The model under review builds one solid part; all positions refer to its coordinate system, in mm. Round coordinates to 2 decimals unless told otherwise and drop trailing zeros. Order: outer loops, then holes, each group sorted by start corner. A loop starts at its lowest first (then second) coordinate and runs counter-clockwise, first axis right, second up. Notation, with made-up numbers: M 74,-39.75 L 92,-39.75 A15 ccw 92,-25.75 Z; hole C 39,-12.5 d8. An arc over 180 degrees is marked long. One line per item, written item: value. Start each with the question number.
from build123d import *
from build123d.topology import SkipClean

# Parameters (mm, degrees)
SKETCH1_R                     = 10.5
SKETCH1_W                     = 8
SKETCH1_H                     = 40
SKETCH1_R_2                   = 5
BOSS_EXTRUDE1_DEPTH           = 3
CUT_EXTRUDE1_REACH            = 140.687
SKETCH2_R                     = 2
BOSS_EXTRUDE2_DEPTH           = 3
SKETCH5_R                     = 2
CUT_EXTRUDE2_DEPTH            = 10
BOSS_EXTRUDE4_START           = -3
BOSS_EXTRUDE4_DEPTH           = 3
BOSS_EXTRUDE5_START           = -3
SKETCH8_R                     = 65
SKETCH8_R_2                   = 10.5
BOSS_EXTRUDE5_DEPTH           = 3
CUT_EXTRUDE4_START            = -10
CUT_EXTRUDE4_DEPTH            = 10
CUT_EXTRUDE6_REACH            = 237.869
SKETCH11_R                    = 2
CUT_EXTRUDE7_REACH            = 237.869
SKETCH12_R                    = 2
CSK_FOR_M3_SFHCS1_D           = 3.4
CSK_FOR_M3_SFHCS1_DEPTH       = 11.3
CSK_FOR_M3_SFHCS1_CSINK_D     = 6.72
CSK_FOR_M3_SFHCS1_CSINK_ANGLE = 90
CSK_FOR_M3_SFHCS1_TIP         = 1.021463052
CSK_FOR_M4_SFHCS1_D           = 4.5
CSK_FOR_M4_SFHCS1_DEPTH       = 11.3
CSK_FOR_M4_SFHCS1_CSINK_D     = 8.96
CSK_FOR_M4_SFHCS1_CSINK_ANGLE = 90
CSK_FOR_M4_SFHCS1_TIP         = 1.351936393
CSK_FOR_M3_SFHCS2_D           = 3.4
CSK_FOR_M3_SFHCS2_DEPTH       = 11.3
CSK_FOR_M3_SFHCS2_CSINK_D     = 6.72
CSK_FOR_M3_SFHCS2_CSINK_ANGLE = 90
CSK_FOR_M3_SFHCS2_TIP         = 1.021463052
CSK_FOR_M4_SFHCS2_D           = 4.5
CSK_FOR_M4_SFHCS2_DEPTH       = 11.3
CSK_FOR_M4_SFHCS2_CSINK_D     = 8.96
CSK_FOR_M4_SFHCS2_CSINK_ANGLE = 90
CSK_FOR_M4_SFHCS2_TIP         = 1.351936393
CUT_EXTRUDE8_REACH            = 237.869
SKETCH23_R                    = 1.5
CSK_FOR_M3_SFHCS3_D           = 3.4
CSK_FOR_M3_SFHCS3_DEPTH       = 11.3
CSK_FOR_M3_SFHCS3_CSINK_D     = 6.72
CSK_FOR_M3_SFHCS3_CSINK_ANGLE = 90
CSK_FOR_M3_SFHCS3_TIP         = 1.021463052


with BuildPart() as part:
    # Sketch1 → Boss-Extrude1 (new body)
    # profile 1 of 2: a face of its own
    with BuildSketch(Plane.XY):
        with BuildLine():
            ThreePointArc((-60, 0), (-52.867640737, 28.372743309), (-33.166247904, 50))
            Line((-33.166247904, 50), (-60, 50))
            Line((-60, 50), (-60, 0))
        make_face()
    # profile 2 of 2: a face of its own
    with BuildSketch(Plane.XY):
        with BuildLine():
            ThreePointArc((0, 60), (-17.320508076, 57.445626465), (-33.166247904, 50))
            ThreePointArc((-33.166247904, 50), (-52.867640737, 28.372743309), (-60, 0))
            ThreePointArc((-60, 0), (-15.529142706, -57.955549577), (51.961524227, -30))
            Line((51.961524227, -30), (56.882127578, -30))
            Line((56.882127578, -30), (90, -30))
            Line((90, -30), (90, -10.355339059))
            Line((90, -10.355339059), (117.67766953, 17.32233047))
            ThreePointArc((117.67766953, 17.32233047), (123.096988313, 44.567085809), (100, 60))
            Line((100, 60), (0, 60))
        make_face()
        Circle(SKETCH1_R, mode=Mode.SUBTRACT)
        with Locations((76, 0)):
            Rectangle(SKETCH1_W, SKETCH1_H, mode=Mode.SUBTRACT)
        with Locations((100, 35)):
            Circle(SKETCH1_R_2, mode=Mode.SUBTRACT)
    extrude(amount=BOSS_EXTRUDE1_DEPTH)

    # Sketch2 → Cut-Extrude1 (cut, up to next)
    with BuildSketch(Plane.XY.offset(3), mode=Mode.PRIVATE) as cut_extrude1_sk1:
        with Locations((60, 45)):
            Circle(SKETCH2_R)
    cut_extrude1_tool1 = extrude(cut_extrude1_sk1.sketch, amount=-CUT_EXTRUDE1_REACH, mode=Mode.PRIVATE) & part.part
    add(cut_extrude1_tool1.solids().sort_by_distance((60, 45, 3))[0], mode=Mode.SUBTRACT)

    # Sketch3 → Boss-Extrude2 (add)
    with BuildSketch(Plane(origin=(0, 0, 0), x_dir=(-1, 0, 0), z_dir=(0, 0, -1))):
        with BuildLine():
            Line((-30, 80), (-30, 60))
            Line((-30, 60), (0, 60))
            ThreePointArc((0, 60), (2.502176759, 59.947803225), (5, 59.791303716))
            Line((5, 59.791303716), (5, 80))
            Line((5, 80), (-30, 80))
        make_face()
    extrude(amount=-BOSS_EXTRUDE2_DEPTH)

    # Sketch5 → Cut-Extrude2 (cut)
    with BuildSketch(Plane.XY.offset(3)):
        with Locations((92, 43)):
            Circle(SKETCH5_R)
        with Locations((108, 43)):
            Circle(SKETCH5_R)
        with Locations((108, 27)):
            Circle(SKETCH5_R)
        with Locations((92, 27)):
            Circle(SKETCH5_R)
    extrude(amount=-CUT_EXTRUDE2_DEPTH, mode=Mode.SUBTRACT)

    # Sketch6 → Boss-Extrude4 (add)
    with BuildSketch(Plane.XY.offset(3).offset(BOSS_EXTRUDE4_START)):
        with BuildLine():
            Line((12.5, 60), (55, 60))
            Line((55, 60), (55, 200))
            Line((55, 200), (-30, 200))
            Line((-30, 200), (-30, 60))
            Line((-30, 60), (-30, 51.961524227))
            ThreePointArc((-30, 51.961524227), (-17.93255034, 57.257520364), (-5, 59.791303716))
            Line((-5, 59.791303716), (-5, 60))
            Line((-5, 60), (12.5, 60))
        make_face()
    extrude(amount=BOSS_EXTRUDE4_DEPTH)

    # Sketch8 → Boss-Extrude5 (add)
    with BuildSketch(Plane.XY.offset(3).offset(BOSS_EXTRUDE5_START)):
        Circle(SKETCH8_R)
        Circle(SKETCH8_R_2, mode=Mode.SUBTRACT)
    extrude(amount=BOSS_EXTRUDE5_DEPTH)

    # Sketch9 → Cut-Extrude4 (cut)
    with SkipClean():  # the faces are left unmerged after this step: merging them gives an invalid solid
        with BuildSketch(Plane.XY.offset(3).offset(CUT_EXTRUDE4_START)):
            with BuildLine():
                Line((-60, 50), (-60, 25))
                ThreePointArc((-60, 25), (-52.282822987, 38.62002616), (-41.533119315, 50))
                Line((-41.533119315, 50), (-60, 50))
            make_face()
        extrude(amount=CUT_EXTRUDE4_DEPTH, mode=Mode.SUBTRACT)

    # Sketch11 → Cut-Extrude6 (cut, up to next)
    with BuildSketch(Plane(origin=(0, 0, 0), x_dir=(-1, 0, 0), z_dir=(0, 0, -1)), mode=Mode.PRIVATE) as cut_extrude6_sk1:
        with Locations((-2.5, 116.34)):
            Circle(SKETCH11_R)
    cut_extrude6_tool1 = extrude(cut_extrude6_sk1.sketch, amount=-CUT_EXTRUDE6_REACH, mode=Mode.PRIVATE) & part.part
    # Sketch11 → Cut-Extrude6 (cut, up to next)
    with BuildSketch(Plane(origin=(0, 0, 0), x_dir=(-1, 0, 0), z_dir=(0, 0, -1)), mode=Mode.PRIVATE) as cut_extrude6_sk2:
        with Locations((-22.5, 116.34)):
            Circle(SKETCH11_R)
    cut_extrude6_tool2 = extrude(cut_extrude6_sk2.sketch, amount=-CUT_EXTRUDE6_REACH, mode=Mode.PRIVATE) & part.part
    add(cut_extrude6_tool1.solids().sort_by_distance((2.5, 116.34, 0))[0], mode=Mode.SUBTRACT)
    add(cut_extrude6_tool2.solids().sort_by_distance((22.5, 116.34, 0))[0], mode=Mode.SUBTRACT)

    # Sketch12 → Cut-Extrude7 (cut, up to next)
    with BuildSketch(Plane(origin=(0, 0, 0), x_dir=(-1, 0, 0), z_dir=(0, 0, -1)), mode=Mode.PRIVATE) as cut_extrude7_sk1:
        with Locations((-2.5, 58.160508076)):
            Circle(SKETCH12_R)
    cut_extrude7_tool1 = extrude(cut_extrude7_sk1.sketch, amount=-CUT_EXTRUDE7_REACH, mode=Mode.PRIVATE) & part.part
    # Sketch12 → Cut-Extrude7 (cut, up to next)
    with BuildSketch(Plane(origin=(0, 0, 0), x_dir=(-1, 0, 0), z_dir=(0, 0, -1)), mode=Mode.PRIVATE) as cut_extrude7_sk2:
        with Locations((-22.5, 58.160508076)):
            Circle(SKETCH12_R)
    cut_extrude7_tool2 = extrude(cut_extrude7_sk2.sketch, amount=-CUT_EXTRUDE7_REACH, mode=Mode.PRIVATE) & part.part
    # Sketch12 → Cut-Extrude7 (cut, up to next)
    with BuildSketch(Plane(origin=(0, 0, 0), x_dir=(-1, 0, 0), z_dir=(0, 0, -1)), mode=Mode.PRIVATE) as cut_extrude7_sk3:
        with Locations((-2.5, 43.160508076)):
            Circle(SKETCH12_R)
    cut_extrude7_tool3 = extrude(cut_extrude7_sk3.sketch, amount=-CUT_EXTRUDE7_REACH, mode=Mode.PRIVATE) & part.part
    # Sketch12 → Cut-Extrude7 (cut, up to next)
    with BuildSketch(Plane(origin=(0, 0, 0), x_dir=(-1, 0, 0), z_dir=(0, 0, -1)), mode=Mode.PRIVATE) as cut_extrude7_sk4:
        with Locations((-22.5, 43.160508076)):
            Circle(SKETCH12_R)
    cut_extrude7_tool4 = extrude(cut_extrude7_sk4.sketch, amount=-CUT_EXTRUDE7_REACH, mode=Mode.PRIVATE) & part.part
    add(cut_extrude7_tool1.solids().sort_by_distance((2.5, 58.160508, 0))[0], mode=Mode.SUBTRACT)
    add(cut_extrude7_tool2.solids().sort_by_distance((22.5, 58.160508, 0))[0], mode=Mode.SUBTRACT)
    add(cut_extrude7_tool3.solids().sort_by_distance((2.5, 43.160508, 0))[0], mode=Mode.SUBTRACT)
    add(cut_extrude7_tool4.solids().sort_by_distance((22.5, 43.160508, 0))[0], mode=Mode.SUBTRACT)

    # CSK for M3 SFHCS1
    with Locations(Plane(origin=(0, 0, 0), x_dir=(-1, 0, 0), z_dir=(0, 0, -1))):
        with Locations((22.5, 38.97114317), (38.97114317, -22.5), (-22.5, -38.97114317), (-96.767766953, 10.554563517)):
            CounterSinkHole(CSK_FOR_M3_SFHCS1_D / 2, CSK_FOR_M3_SFHCS1_CSINK_D / 2, depth=CSK_FOR_M3_SFHCS1_DEPTH, counter_sink_angle=CSK_FOR_M3_SFHCS1_CSINK_ANGLE)
            with Locations((0, 0, -(CSK_FOR_M3_SFHCS1_DEPTH + CSK_FOR_M3_SFHCS1_TIP / 2))):  # 118° drill point
                Cone(0, CSK_FOR_M3_SFHCS1_D / 2, CSK_FOR_M3_SFHCS1_TIP, mode=Mode.SUBTRACT)

    # CSK for M4 SFHCS1
    with Locations(Plane(origin=(0, 0, 0), x_dir=(-1, 0, 0), z_dir=(0, 0, -1))):
        with Locations((-49, 194.5), (24, 194.5), (24, 130), (-49, 130), (-49, 65.5), (24, 65.5)):
            CounterSinkHole(CSK_FOR_M4_SFHCS1_D / 2, CSK_FOR_M4_SFHCS1_CSINK_D / 2, depth=CSK_FOR_M4_SFHCS1_DEPTH, counter_sink_angle=CSK_FOR_M4_SFHCS1_CSINK_ANGLE)
            with Locations((0, 0, -(CSK_FOR_M4_SFHCS1_DEPTH + CSK_FOR_M4_SFHCS1_TIP / 2))):  # 118° drill point
                Cone(0, CSK_FOR_M4_SFHCS1_D / 2, CSK_FOR_M4_SFHCS1_TIP, mode=Mode.SUBTRACT)

    # CSK for M3 SFHCS2
    with Locations(Plane(origin=(0, 0, 0), x_dir=(-1, 0, 0), z_dir=(0, 0, -1))):
        with Locations((-83, -26), (-69, -26)):
            CounterSinkHole(CSK_FOR_M3_SFHCS2_D / 2, CSK_FOR_M3_SFHCS2_CSINK_D / 2, depth=CSK_FOR_M3_SFHCS2_DEPTH, counter_sink_angle=CSK_FOR_M3_SFHCS2_CSINK_ANGLE)
            with Locations((0, 0, -(CSK_FOR_M3_SFHCS2_DEPTH + CSK_FOR_M3_SFHCS2_TIP / 2))):  # 118° drill point
                Cone(0, CSK_FOR_M3_SFHCS2_D / 2, CSK_FOR_M3_SFHCS2_TIP, mode=Mode.SUBTRACT)

    # CSK for M4 SFHCS2
    with Locations(Plane(origin=(0, 0, 0), x_dir=(-1, 0, 0), z_dir=(0, 0, -1))):
        with Locations((-60, 45)):
            CounterSinkHole(CSK_FOR_M4_SFHCS2_D / 2, CSK_FOR_M4_SFHCS2_CSINK_D / 2, depth=CSK_FOR_M4_SFHCS2_DEPTH, counter_sink_angle=CSK_FOR_M4_SFHCS2_CSINK_ANGLE)
            with Locations((0, 0, -(CSK_FOR_M4_SFHCS2_DEPTH + CSK_FOR_M4_SFHCS2_TIP / 2))):  # 118° drill point
                Cone(0, CSK_FOR_M4_SFHCS2_D / 2, CSK_FOR_M4_SFHCS2_TIP, mode=Mode.SUBTRACT)

    # Sketch23 → Cut-Extrude8 (cut, up to next)
    with BuildSketch(Plane(origin=(0, 0, 0), x_dir=(-1, 0, 0), z_dir=(0, 0, -1)), mode=Mode.PRIVATE) as cut_extrude8_sk1:
        with Locations((-79.5, 35)):
            Circle(SKETCH23_R)
    cut_extrude8_tool1 = extrude(cut_extrude8_sk1.sketch, amount=-CUT_EXTRUDE8_REACH, mode=Mode.PRIVATE) & part.part
    # Sketch23 → Cut-Extrude8 (cut, up to next)
    with BuildSketch(Plane(origin=(0, 0, 0), x_dir=(-1, 0, 0), z_dir=(0, 0, -1)), mode=Mode.PRIVATE) as cut_extrude8_sk2:
        with Locations((-110.25, 17.246479222)):
            Circle(SKETCH23_R)
    cut_extrude8_tool2 = extrude(cut_extrude8_sk2.sketch, amount=-CUT_EXTRUDE8_REACH, mode=Mode.PRIVATE) & part.part
    # Sketch23 → Cut-Extrude8 (cut, up to next)
    with BuildSketch(Plane(origin=(0, 0, 0), x_dir=(-1, 0, 0), z_dir=(0, 0, -1)), mode=Mode.PRIVATE) as cut_extrude8_sk3:
        with Locations((-110.25, 52.753520778)):
            Circle(SKETCH23_R)
    cut_extrude8_tool3 = extrude(cut_extrude8_sk3.sketch, amount=-CUT_EXTRUDE8_REACH, mode=Mode.PRIVATE) & part.part
    add(cut_extrude8_tool1.solids().sort_by_distance((79.5, 35, 0))[0], mode=Mode.SUBTRACT)
    add(cut_extrude8_tool2.solids().sort_by_distance((110.25, 17.246479, 0))[0], mode=Mode.SUBTRACT)
    add(cut_extrude8_tool3.solids().sort_by_distance((110.25, 52.753521, 0))[0], mode=Mode.SUBTRACT)

    # CSK for M3 SFHCS3
    with Locations(Plane(origin=(0, 0, 0), x_dir=(-1, 0, 0), z_dir=(0, 0, -1))):
        with Locations((-44, 0)):
            CounterSinkHole(CSK_FOR_M3_SFHCS3_D / 2, CSK_FOR_M3_SFHCS3_CSINK_D / 2, depth=CSK_FOR_M3_SFHCS3_DEPTH, counter_sink_angle=CSK_FOR_M3_SFHCS3_CSINK_ANGLE)
            with Locations((0, 0, -(CSK_FOR_M3_SFHCS3_DEPTH + CSK_FOR_M3_SFHCS3_TIP / 2))):  # 118° drill point
                Cone(0, CSK_FOR_M3_SFHCS3_D / 2, CSK_FOR_M3_SFHCS3_TIP, mode=Mode.SUBTRACT)


solid = part.part
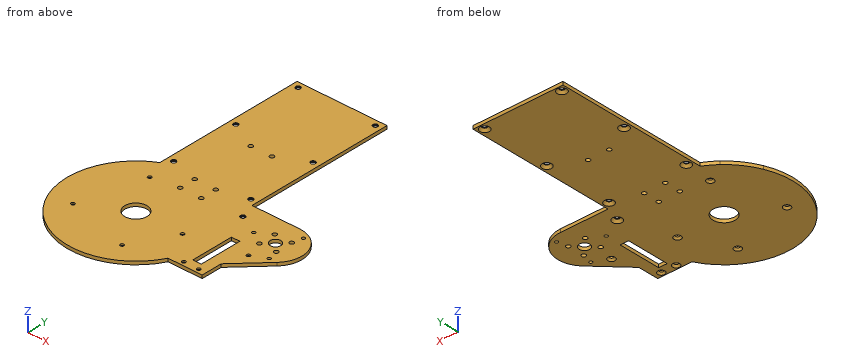
Item 1: Wall thickness on L1, parallel to X at y = 65.5, z = 2.6; L2, parallel to Y at x = 92, z = 1.9; L3, parallel to Y at x = 79, z = 0.2: over which ranges is each line inside the solid? List them lowest first.
Item 2: Consider section B-B, the plane z = 0.55. Count the separate pieces of the cut face and the enclosed holes in it, then the cut area to 3 significant figures.
Item 3: Consider section C-C, the plane x = -45. Give the boundary of the cut face in (y, z).
Item 4: Consider section A-A, the plane y = 94. Give the boundary of the cut face in (x, z), then the cut area to 3 significant figures.
Item 5: Clearance check with flat-ended pins moving along their axes: P1, Ø1.5, axis at y = 144.5, z = 1, coming from the -X side; P2, Ø5, axis at x = -24, y = 194.5, coming from the +Z side; P3, Ø5, axis at x = 60, y = 45, coming from the -Z side; P4, Ø0.9, axis at x = 85, z = 1.5, coming from the +Y side. State where each tip first meets the part, or that it passes through.
Computed:
1. L1: x = -30 to -26.25, -21.75 to 46.75, 51.25 to 55
1. L2: y = -8.36 to 25, 29 to 41, 45 to 60
1. L3: y = -30 to -20, 20 to 33.59, 36.41 to 60
2. separate pieces: 1
2. enclosed holes: 30
2. area: 28,300 mm^2
3. outline: M -46.9,0 L 46.9,0 L 46.9,3 L -46.9,3 Z
4. outline: M -30,0 L 55,0 L 55,3 L -30,3 Z
4. area: 255 mm^2
5. P1: stops at x = -30
5. P2: stops at z = 3
5. P3: stops at z = 1.98
5. P4: stops at y = 60
